Could you check a few things on this model? Use its own coordinates, in mm. Round coordinates to 2 decimals unless told otherwise and drop trailing zeros. Loops run counter-clockwise (first coordinate to the right, second up) from the corner with the lowest first, then second, coordinate; pieces in that order, holes last. Notation, with made-up numbers: (-39, -4) -> (-31, -4) arc R14 ccw to (-31, 19) -> close; hole circle Ø10 at (57, 16.5). An arc over 180 degrees is marked (long way). Write each question's results on one line, items separated by ' | '.
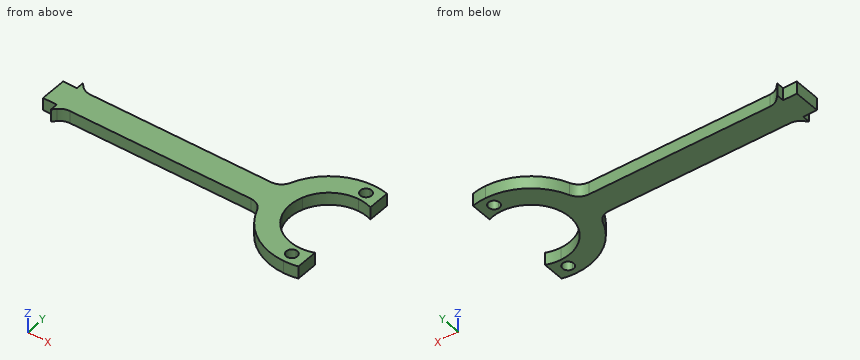
from build123d import *

# Parameters (mm, degrees)
F0_W     = 5
F0_H     = 9.5
F1_DEPTH = 4.5
F2_R     = 5


with BuildPart() as f1:
    # F0 (on Top) → F1 (new body)
    with BuildSketch(Plane.XY):
        with Locations((-47.5, 0)):
            Rectangle(F0_W, F0_H)
        with BuildLine():
            Line((36.8304328089, 4.75), (29.0312732862, 4.75))
            ThreePointArc((29.0312732862, 4.75), (28.5, 0), (29.0312732862, -4.75))
            Line((29.0312732862, -4.75), (36.8304328089, -4.75))
            ThreePointArc((36.8304328089, -4.75), (36, 0), (36.8304328089, 4.75))
        make_face()
        with BuildLine():
            ThreePointArc((50, 21.5), (36.5812630997, 16.7984374273), (29.0312732862, 4.75))
            Line((29.0312732862, 4.75), (36.8304328089, 4.75))
            ThreePointArc((36.8304328089, 4.75), (41.9532615303, 11.4564392374), (50, 14))
            Line((50, 14), (50, 15.5))
            ThreePointArc((50, 15.5), (48, 17.5), (50, 19.5))
            Line((50, 19.5), (50, 21.5))
        make_face()
        with BuildLine():
            Line((36.8304328089, -4.75), (29.0312732862, -4.75))
            ThreePointArc((29.0312732862, -4.75), (36.5812630997, -16.7984374273), (50, -21.5))
            Line((50, -21.5), (50, -19.5))
            ThreePointArc((50, -19.5), (48, -17.5), (50, -15.5))
            Line((50, -15.5), (50, -14))
            ThreePointArc((50, -14), (41.9532615303, -11.4564392374), (36.8304328089, -4.75))
        make_face()
        with BuildLine():
            Line((50, -19.5), (50, -21.5))
            ThreePointArc((50, -21.5), (52.5173141614, -21.3521223632), (55, -20.9105236663))
            Line((55, -20.9105236663), (55, -13.0766968306))
            ThreePointArc((55, -13.0766968306), (52.542267135, -13.7672392953), (50, -14))
            Line((50, -14), (50, -15.5))
            ThreePointArc((50, -15.5), (51.4142135624, -16.0857864376), (52, -17.5))
            ThreePointArc((52, -17.5), (51.4142135624, -18.9142135624), (50, -19.5))
        make_face()
        with BuildLine():
            ThreePointArc((55, 20.9105236663), (52.5173141614, 21.3521223632), (50, 21.5))
            Line((50, 21.5), (50, 19.5))
            ThreePointArc((50, 19.5), (51.4142135624, 18.9142135624), (52, 17.5))
            ThreePointArc((52, 17.5), (51.4142135624, 16.0857864376), (50, 15.5))
            Line((50, 15.5), (50, 14))
            ThreePointArc((50, 14), (52.542267135, 13.7672392953), (55, 13.0766968306))
            Line((55, 13.0766968306), (55, 20.9105236663))
        make_face()
        with BuildLine():
            Line((29.0312732862, 4.75), (-42.25, 4.75))
            Line((-42.25, 4.75), (-37.5, 0))
            Line((-37.5, 0), (-42.25, -4.75))
            Line((-42.25, -4.75), (29.0312732862, -4.75))
            ThreePointArc((29.0312732862, -4.75), (28.5, 0), (29.0312732862, 4.75))
        make_face()
        Polygon((-42.25, 4.75), (-45, 4.75), (-45, -4.75), (-42.25, -4.75), (-37.5, 0), align=None)
        Polygon((-45, 7.5), (-45, 4.75), (-42.25, 4.75), align=None)
        Polygon((-42.25, -4.75), (-45, -4.75), (-45, -7.5), align=None)
    extrude(amount=F1_DEPTH)

    # F2
    f2_edges = [f1.edges().sort_by_distance(p)[0] for p in [
        (29.031273, -4.75, 2.25),
        (29.031273, 4.75, 2.25),
        (-42.25, -4.75, 2.25),
        (-42.25, 4.75, 2.25),
    ]]
    fillet(f2_edges, radius=F2_R)


solid = f1.part
1) I'm going to push flat-ended pins straight in: pin 1 (2 mm diameter, centred on x = -47.5, z = 2, fed in from -Y); pin 2 (1 mm diameter, centred on x = -16.5, z = 1.5, fed in from +Y); pin 3 (1 mm diameter, centred on y = 2.5, z = 3.5, fed in from +X). Where does each tip first touch, or does it pass through?
Model answer:
pin 1: stops at y = -4.75 | pin 2: stops at y = 4.75 | pin 3: stops at x = 36.33
2) I want a section at B-B, the plane x = -13. Write out the boundary of the cut face in (y, z), plus the area to 4 significant figures.
Model answer:
outline: (-4.75, 0) -> (4.75, 0) -> (4.75, 4.5) -> (-4.75, 4.5) -> close | area: 42.75 mm2
3) I want a section at A-A, the plane z = 3.25. Write out the boundary of the cut face in (x, y).
Model answer:
outline: (-50, -4.75) -> (-45, -4.75) -> (-45, -7.5) -> (-43.71, -6.21) arc R5 cw to (-40.18, -4.75) -> (25.36, -4.75) arc R5 cw to (30.01, -7.91) arc R21.5 ccw to (55, -20.91) -> (55, -13.08) arc R14 cw (long way) to (55, 13.08) -> (55, 20.91) arc R21.5 ccw to (30.01, 7.91) arc R5 cw to (25.36, 4.75) -> (-40.18, 4.75) arc R5 cw to (-43.71, 6.21) -> (-45, 7.5) -> (-45, 4.75) -> (-50, 4.75) -> close; hole circle Ø4 at (50, -17.5); hole circle Ø4 at (50, 17.5)
4) I need wall thicknesses on line 1 (Y direction, x = 15, z = 3.1); line 2 (X direction, y = -17, z = 2.3); line 3 (Y direction, x = 42, z = 0.55). Which ranges of each line are inside material? Lowest first, please.
Model answer:
line 1: y = -4.75 to 4.75 | line 2: x = 36.84 to 48.06, 51.94 to 55 | line 3: y = -19.96 to -11.49, 11.49 to 19.96
